Drawing for the job (mm, zero at the part's lowest x, y, z). Coordinates: 2 decimals unless noted, no trailing zeros. Write each loop counter-clockwise with the first axis right and the second up, starting at its lowest first coordinate (ties: lowest second). Pieces come first, ordered by that corner, then holes. Notation, with made-up numbers: (85, 79.25) -> (112, 79.25) arc R14 ccw to (112, 87.25) -> close; hole circle Ø4 at (-31, 11.25). An arc over 180 degrees is marked (long way). Write item = value, one per line. Start each with the question number.
Q1. Probe line 1 (X direction, y = 52.5, z = 17.5); line 2 (Y direction, x = 12.5, z = 28.5); line 3 (Y direction, x = 69.5, z = 94). List the from-to ranges inside material, lowest first.
Q2. Band-saw the part on C-C, the plane x = 44. List the corners of the cut face in (y, z).
Q3. Pin check, flat tips, straight feed: P1, Ø3, axis at x = 33, z = 77.5, coming from the +Y side; P2, Ø8, axis at y = 5, z = 54.5, coming from the +X side; P3, Ø3, axis at x = 52, y = 6, coming from the -Z side. Stop position of each tip, or through.
Q4. Band-saw the part on D-D, the plane z = 39. List the corners of the cut face in (x, y), plus the area to 3 significant figures.
Q5. Band-saw the part on A-A, the plane y = 83.5. List the corners of the cut face in (x, z).
Q6. Band-saw the part on B-B, the plane z = 93.5. List the corners of the cut face in (x, y), plus the area to 3 significant figures.
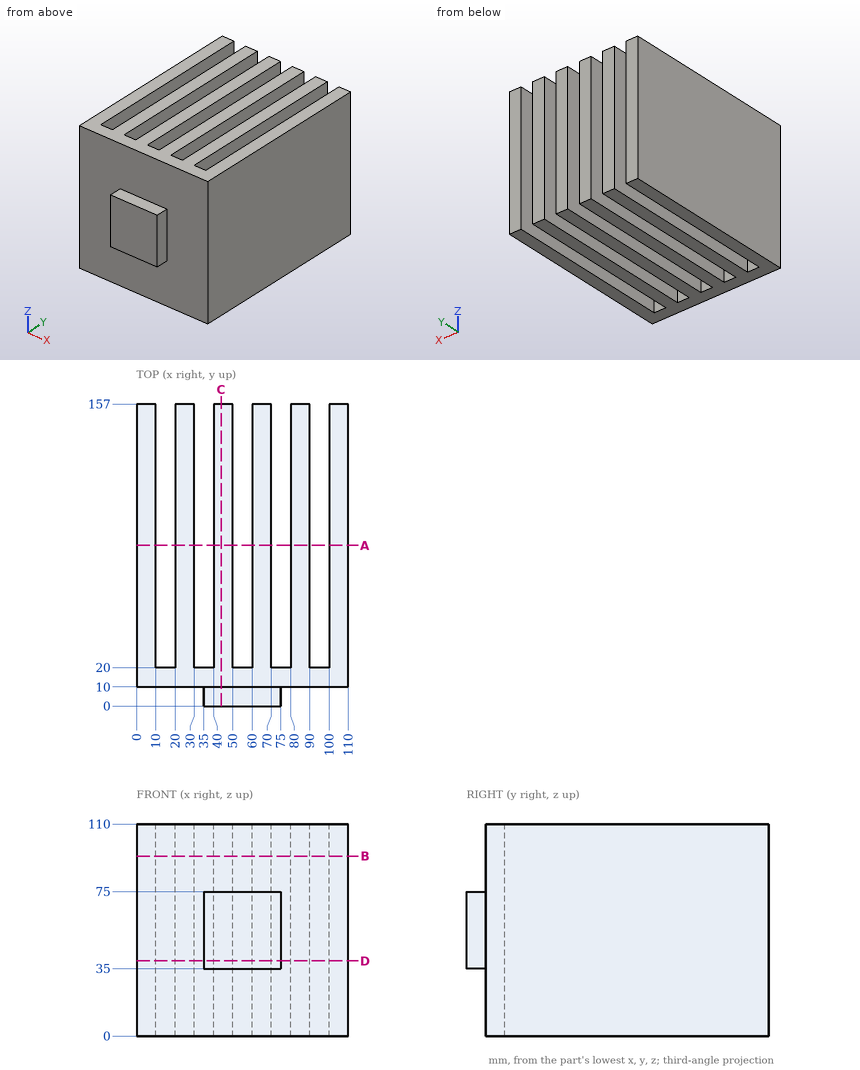
Ans:
q1.line_1 = 0 to 10, 20 to 30, 40 to 50, 60 to 70, 80 to 90, 100 to 110
q1.line_2 = 10 to 20
q1.line_3 = 10 to 157
q2.outline = (0, 35) -> (10, 35) -> (10, 0) -> (157, 0) -> (157, 110) -> (10, 110) -> (10, 75) -> (0, 75) -> close
q3.P1 = 20
q3.P2 = 75
q3.P3 = 35
q4.outline = (0, 10) -> (35, 10) -> (35, 0) -> (75, 0) -> (75, 10) -> (110, 10) -> (110, 157) -> (100, 157) -> (100, 20) -> (90, 20) -> (90, 157) -> (80, 157) -> (80, 20) -> (70, 20) -> (70, 157) -> (60, 157) -> (60, 20) -> (50, 20) -> (50, 157) -> (40, 157) -> (40, 20) -> (30, 20) -> (30, 157) -> (20, 157) -> (20, 20) -> (10, 20) -> (10, 157) -> (0, 157) -> close
q4.area = 9,720 mm2
q5.outline = (0, 0) -> (10, 0) -> (10, 110) -> (0, 110) -> close; (20, 0) -> (30, 0) -> (30, 110) -> (20, 110) -> close; (40, 0) -> (50, 0) -> (50, 110) -> (40, 110) -> close; (60, 0) -> (70, 0) -> (70, 110) -> (60, 110) -> close; (80, 0) -> (90, 0) -> (90, 110) -> (80, 110) -> close; (100, 0) -> (110, 0) -> (110, 110) -> (100, 110) -> close
q6.outline = (0, 10) -> (110, 10) -> (110, 157) -> (100, 157) -> (100, 20) -> (90, 20) -> (90, 157) -> (80, 157) -> (80, 20) -> (70, 20) -> (70, 157) -> (60, 157) -> (60, 20) -> (50, 20) -> (50, 157) -> (40, 157) -> (40, 20) -> (30, 20) -> (30, 157) -> (20, 157) -> (20, 20) -> (10, 20) -> (10, 157) -> (0, 157) -> close
q6.area = 9,320 mm2
